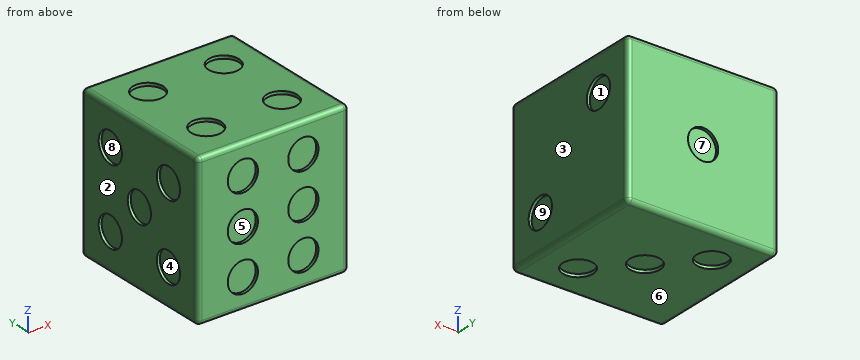
Autodesk Fusion 360 part; units mm, degrees
sketch "Sketch1" plane through (0, 0, 0) normal (0, 1, 0) x (1, 0, 0)
  line L0 (0, 0) -> (10, 0)
  line L1 (10, 0) -> (10, -10)
  line L2 (10, -10) -> (0, -10)
  line L3 (0, -10) -> (0, 0)
  dimension "d1" = 10
  dimension "d2" = 10
extrude "Extrude1" add sketch "Sketch1" along normal blind 10
sketch "Sketch2" plane through (0, 10, 0) normal (0, 1, 0) x (-1, 0, 0)
  line L0 (0, 10) -> (-10, 10)
  line L1 (-10, 10) -> (-10, 0)
  line L2 (-10, 0) -> (0, 0)
  line L3 (0, 0) -> (0, 10)
  circle A0 centre (-5, 5) radius 1
  dimension "d5" = 2
  dimension "d24" = 5
  dimension "d25" = 5
sketch "Sketch3" plane through (0, 0, 0) normal (0, -1, 0) x (1, 0, 0)
  line L0 (10, 10) -> (0, 10)
  line L1 (0, 10) -> (0, 0)
  line L2 (0, 0) -> (10, 0)
  line L3 (10, 0) -> (10, 10)
  circle A0 centre (3, 8) radius 1
  circle A1 centre (3, 5) radius 1
  circle A2 centre (3, 2) radius 1
  circle A3 centre (7, 8) radius 1
  circle A4 centre (7, 5) radius 1
  circle A5 centre (7, 2) radius 1
  dimension "d6" = 2
  dimension "d7" = 2
  dimension "d8" = 2
  dimension "d9" = 2
  dimension "d10" = 2
  dimension "d11" = 2
  dimension "d12" = 3
  dimension "d13" = 3
  dimension "d14" = 3
  dimension "d15" = 3
  dimension "d16" = 3
  dimension "d17" = 3
  dimension "d18" = 3
  dimension "d19" = 3
  dimension "d20" = 2
  dimension "d21" = 2
  dimension "d22" = 3
  dimension "d23" = 3
sketch "Sketch4" plane through (0, 0, 0) normal (-1, 0, 0) x (0, 0, 1)
  line L0 (0, 0) -> (10, 0)
  line L1 (10, 0) -> (10, 10)
  line L2 (10, 10) -> (0, 10)
  line L3 (0, 10) -> (0, 0)
  circle A0 centre (7.5, 2.5) radius 1
  circle A1 centre (5, 5) radius 1
  circle A2 centre (2.5, 7.5) radius 1
  circle A3 centre (2.5, 2.5) radius 1
  circle A4 centre (7.5, 7.5) radius 1
  line L4 (10, 0) -> (0, 0)
  line L5 (0, 10) -> (10, 10)
  dimension "d26" = 2
  dimension "d27" = 2
  dimension "d28" = 2
  dimension "d29" = 2
  dimension "d30" = 2
  dimension "d31" = 2.5
  dimension "d32" = 2.5
  dimension "d33" = 2.5
  dimension "d34" = 2.5
  dimension "d35" = 2.5
  dimension "d36" = 2.5
  dimension "d37" = 2.5
  dimension "d38" = 2.5
  dimension "d39" = 5
  dimension "d40" = 5
sketch "Sketch5" plane through (0, 0, 0) normal (0, 0, -1) x (-1, 0, 0)
  line L0 (-10, 0) -> (0, 0)
  line L1 (0, 0) -> (0, 10)
  line L2 (0, 10) -> (-10, 10)
  line L3 (-10, 10) -> (-10, 0)
  circle A0 centre (-5, 5) radius 1
  circle A1 centre (-7.5, 2.5) radius 1
  circle A2 centre (-2.5, 7.5) radius 1
  line L4 (0, 10) -> (0, 0)
  line L5 (-10, 10) -> (0, 10)
  line L6 (0, 0) -> (-10, 0)
  dimension "d41" = 2
  dimension "d42" = 2
  dimension "d43" = 2
  dimension "d44" = 2.5
  dimension "d45" = 2.5
  dimension "d46" = 2.5
  dimension "d47" = 2.5
  dimension "d48" = 5
  dimension "d49" = 5
sketch "Sketch6" plane through (10, 0, 0) normal (1, 0, 0) x (0, 0, -1)
  line L0 (-10, 0) -> (0, 0)
  line L1 (0, 0) -> (0, 10)
  line L2 (0, 10) -> (-10, 10)
  line L3 (-10, 10) -> (-10, 0)
  circle A0 centre (-2.5, 2.5) radius 1
  circle A1 centre (-7.5, 7.5) radius 1
  line L4 (0, 0) -> (-10, 0)
  line L5 (-10, 10) -> (0, 10)
  dimension "d50" = 2
  dimension "d51" = 2
  dimension "d52" = 2.5
  dimension "d53" = 2.5
  dimension "d54" = 2.5
  dimension "d55" = 2.5
sketch "Sketch7" plane through (0, 0, 10) normal (0, 0, 1) x (1, 0, 0)
  line L0 (0, 0) -> (10, 0)
  line L1 (10, 0) -> (10, 10)
  line L2 (10, 10) -> (0, 10)
  line L3 (0, 10) -> (0, 0)
  circle A0 centre (7.5, 2.5) radius 1
  circle A1 centre (2.5, 7.5) radius 1
  circle A2 centre (2.5, 2.5) radius 1
  circle A3 centre (7.5, 7.5) radius 1
  line L4 (10, 0) -> (0, 0)
  line L5 (0, 0) -> (0, 10)
  line L6 (10, 10) -> (10, 0)
  dimension "d56" = 2
  dimension "d57" = 2
  dimension "d58" = 2
  dimension "d59" = 2
  dimension "d60" = 2.5
  dimension "d61" = 2.5
  dimension "d62" = 2.5
  dimension "d63" = 2.5
  dimension "d64" = 2.5
  dimension "d65" = 2.5
  dimension "d66" = 2.5
  dimension "d67" = 2.5
extrude "Extrude2" cut sketch "Sketch3" against normal blind 0.2 contours A0 | A1 | A2 | A3 | A4 | A5
extrude "Extrude3" cut sketch "Sketch7" against normal blind 0.2 contours A0 | A1 | A2 | A3
extrude "Extrude4" cut sketch "Sketch4" against normal blind 0.2 contours A0 | A1 | A2 | A3 | A4
extrude "Extrude5" cut sketch "Sketch6" against normal blind 0.2 contours A0 | A1
extrude "Extrude6" cut sketch "Sketch5" against normal blind 0.2 contours A0 | A1 | A2
extrude "Extrude7" cut sketch "Sketch2" against normal blind 0.2 contours A0
fillet "Fillet1" radius 0.3 12 edges at (0, 0, 5) (5, 0, 0) (0, 5, 0) (10, 0, 5) (10, 5, 0) (5, 10, 0) (10, 10, 5) (10, 5, 10) (5, 0, 10) (0, 5, 10) (0, 10, 5) (5, 10, 10)
Model file for the job. Use its own axes, mm. Face numbers are marked on the shaded views. A direction names the side the tool comes from. Round coordinates to 2 decimals unless told otherwise and drop trailing zeros. Write each loop counter-clockwise with the first axis right and the second up, starting at its lowest first coordinate (ties: lowest second). Pieces come first, ordered by that corner, then holes. Notation, with made-up numbers: M 60,39 L 114,39 A10 cw 114,53 Z; hole C 86,63 d4. An arc over 180 degrees is marked long. Put each result on its own line as item: value.
Item 1: Cut at D-D (z = 2). List the corners of the cut face in (x, y).
Responses:
outline: M 0,0.3 A0.3 ccw 0.3,0 L 2,0 L 2,0.2 L 4,0.2 L 4,0 L 6,0 L 6,0.2 L 8,0.2 L 8,0 L 9.7,0 A0.3 ccw 10,0.3 L 10,1.63 L 9.8,1.63 L 9.8,3.37 L 10,3.37 L 10,9.7 A0.3 ccw 9.7,10 L 0.3,10 A0.3 ccw 0,9.7 L 0,8.37 L 0.2,8.37 L 0.2,6.63 L 0,6.63 L 0,3.37 L 0.2,3.37 L 0.2,1.63 L 0,1.63 Z
Item 2: Cut at A-A (z = 5). List the corners of the cut face in (x, y).
Responses:
outline: M 0,0.3 A0.3 ccw 0.3,0 L 2,0 L 2,0.2 L 4,0.2 L 4,0 L 6,0 L 6,0.2 L 8,0.2 L 8,0 L 9.7,0 A0.3 ccw 10,0.3 L 10,9.7 A0.3 ccw 9.7,10 L 6,10 L 6,9.8 L 4,9.8 L 4,10 L 0.3,10 A0.3 ccw 0,9.7 L 0,6 L 0.2,6 L 0.2,4 L 0,4 Z
Item 3: Flat gauge pins, fed straight in: P1, Ø1, axis at x = 1.5, z = 3.5, coming from the -Y side; P2, Ø1.6, axis at x = 7.5, y = 2.5, coming from the -Z side; P3, Ø1.2, axis at x = 3, z = 2, coming from the -Y side; P4, Ø0.6, axis at y = 7.5, z = 7.5, coming from the +X side. Where does each tip first touch, or does it go through?
Responses:
P1: y = 0
P2: z = 0.2
P3: y = 0.2
P4: x = 9.8
Item 4: Probe L1, parallel to Y at x = 3.25, z = 4.25; L2, parallel to Y at x = 0.1, z = 7.5. List the from-to ranges inside material, lowest first. Write a range as from..to.
Responses:
L1: 0.2..10
L2: 0.08..1.5, 3.5..6.5, 8.5..9.92
Item 5: Tool access for the marked faces 1, 2, 3, 4 and 5: list every direction of +Z, -Z, +X, -X, +Y, -Y with a clear straight run to the whole face (end or side of a thin tool).
Responses:
face 1: +X
face 2: +Z, -Z, -X, +Y, -Y
face 3: +Z, -Z, +X, +Y, -Y
face 4: -X
face 5: -Y
Item 6: Mould opens along X. For the marked faces 6, 7, 8 and 9 say: +X half, -X half, draft (parallel to the pull), parting line (faces both ways), or undercut.
Responses:
face 6: draft
face 7: undercut
face 8: -X half
face 9: +X half
